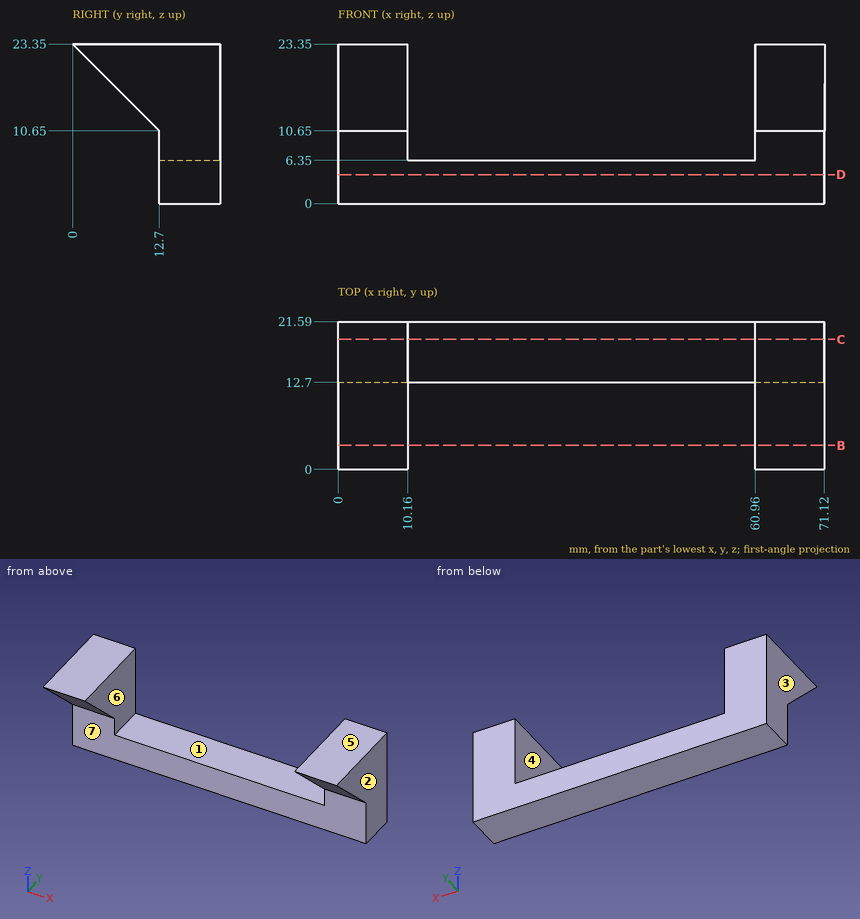
Answer from the drawing. Dimensions are ordinates in mm from the lowest x, y and z of the part. A direction names the side the tool comes from. Coordinates: 2 decimals unless noted, no trailing zeros. Write each loop counter-clockwise with the first axis right and the second up, starting at its lowest first coordinate (ties: lowest second). Pieces come first, ordered by that corner, then holes. Notation, with made-up numbers: (66.5, -33.5) -> (89.5, -33.5) arc R15 cw to (89.5, -5.5) -> close; hole circle Ø10 at (29, 85.5). An arc over 180 degrees is marked (long way). One line per question, with ' | ' between items.
1. Straight lines are drawn through the part: line 1 (X direction, y = 9.5, z = 22.25); line 2 (Y direction, x = 50, z = 2.5); line 3 (Z direction, x = 27, y = 15). For each, find the intervals that lie inside material, in ascending order.
Verdict:
line 1: x = 0 to 10.16, 60.96 to 71.12 | line 2: y = 12.7 to 21.59 | line 3: z = 0 to 6.35
2. Which of the six approach directions +Z, -Z, +X, -X, +Y, -Y give full straight-line access (tool end or side, diameter ignored) to the marked faces 5, 6 and 7?
Verdict:
face 5: +Z, +X, -X, +Y, -Y | face 6: +Z, +Y, -Y | face 7: -Z, +X, -X, -Y
3. Section D-D (z = 4.25) is taken. Determine the outline of the cut face in (x, y), and give its area (3 significant figures).
Verdict:
outline: (0, 12.7) -> (71.12, 12.7) -> (71.12, 21.59) -> (0, 21.59) -> close | area: 632 mm^2
4. Section C-C (y = 19) is taken. Determine the outline of the cut face in (x, z), and give its area (3 significant figures).
Verdict:
outline: (0, 0) -> (71.12, 0) -> (71.12, 23.35) -> (60.96, 23.35) -> (60.96, 6.35) -> (10.16, 6.35) -> (10.16, 23.35) -> (0, 23.35) -> close | area: 797 mm^2
5. Given pin 1 Ø11.5 at (x, z) = (36, 3) entering from -Y; pin 2 Ø2.5 at (x, y) = (35.5, 17.5) entering from +Z; pin 3 Ø8 at (x, y) = (25, 13) entering from -Z; pin 4 Ø12 at (x, z) = (26.5, 14.5) entering from +Y, each flat-ended and moving along its own axis, determine where each tip first touches the part or whether it passes through.
Verdict:
pin 1: stops at y = 12.7 | pin 2: stops at z = 6.35 | pin 3: stops at z = 0 | pin 4: passes through
6. For a pull along X with two mould halves and no side action, classify the marked faces 1, 2, 3 and 4 as released by +X, released by -X, zero draft, split by the parting line, or undercut.
Verdict:
face 1: undercut | face 2: released by +X | face 3: released by -X | face 4: undercut
7. Section B-B (y = 3.5) is taken. Determine the outline of the cut face in (x, z), and give its area (3 significant figures).
Verdict:
outline: (0, 19.85) -> (10.16, 19.85) -> (10.16, 23.35) -> (0, 23.35) -> close; (60.96, 19.85) -> (71.12, 19.85) -> (71.12, 23.35) -> (60.96, 23.35) -> close | area: 71.1 mm^2
